Verification items for the finished model (mm, model axes). Face numbers are marked on the shaded views. A direction names the side the tool comes from. Coordinates: 2 decimals unless noted, no trailing zeros. Loops run counter-clockwise (first coordinate to the right, second up) from the corner with the lowest first, then second, coordinate; pieces in that order, holes last. Notation, with made-up numbers: (20, -32) -> (71, -32) arc R31 ccw to (71, -4) -> close; hole circle Ø8 at (42, 53.5). An arc over 180 degrees is marked (long way). Write item = value, one per line.
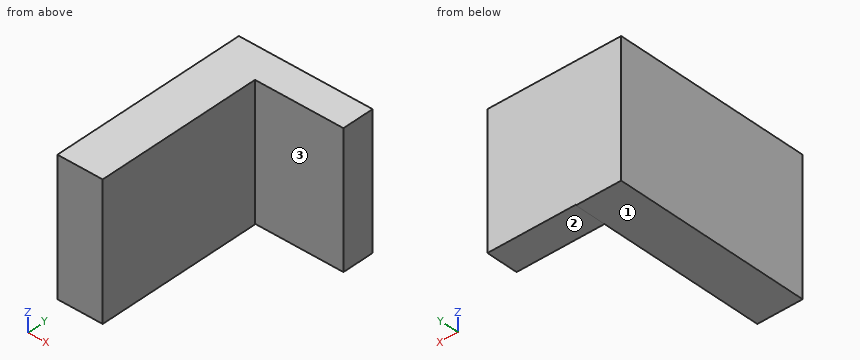
```python
from build123d import *

# Parameters (mm, degrees)
F0_W     = 41.935582
F0_H     = 41.549082
F1_DEPTH = 10
F3_DEPTH = 14.2


with BuildPart() as f1:
    # F0 (on Front) → F1 (new body)
    with BuildSketch(Plane.XZ):
        with Locations((-43.771474, 27.44172)):
            Rectangle(F0_W, F0_H)
    extrude(amount=F1_DEPTH)

    # F2 (on face) → F3 (join)
    with BuildSketch(Plane(origin=(-64.739265, 0, 0), x_dir=(0, -1, 0), z_dir=(-1, 0, 0))):
        Polygon((62.226996, 48.216261), (10, 48.216261), (10, 6.667179), (0, 6.667179), (0, 6.473927), (62.226996, 6.473927), align=None)
    extrude(amount=-F3_DEPTH)


solid = f1.part
```
1) Sectioned sample at A-A, the plane z = 23. Record the cut outline in (x, y).
Ans:
outline = (-64.74, -62.23) -> (-50.54, -62.23) -> (-50.54, -10) -> (-22.8, -10) -> (-22.8, 0) -> (-64.74, 0) -> close
2) Material ranges on line 1 (X direction, y = -47, z = 44.5); line 2 (Y direction, x = -25.5, z = 27), recorded low to high.
Ans:
line_1 = -64.74 to -50.54
line_2 = -10 to 0
3) Depth check by flat-ended pin: pin 1 Ø12 at (x, y) = (-28, -11) entering from -Z; pin 2 Ø6 at (y, z) = (-43.5, 22) entering from +X; pin 3 Ø1.5 at (x, z) = (-38, 17.5) entering from +Y. Enter the tip coordinate at first touch or a pass-through.
Ans:
pin_1 = 6.67
pin_2 = -50.54
pin_3 = 0
4) Tool access check on the marked faces 1, 2 and 3. Record the directions out of +Z, -Z, +X, -X, +Y, -Y that give a thin tool (end or side, any length) a straight path to the whole face; none if there is none.
Ans:
face_1 = -Z, +X, -X, +Y, -Y
face_2 = -Z, +X, +Y, -Y
face_3 = +Z, -Z, +X, -Y
5) Sectioned sample at B-B, the plane x = -28. Record the cut outline in (y, z), plus the area to 3 significant figures.
Ans:
outline = (-10, 6.67) -> (0, 6.67) -> (0, 48.22) -> (-10, 48.22) -> close
area = 415 mm2
6) Sectioned sample at C-C, the plane y = -21. Record the cut outline in (x, z), plus the area to 3 significant figures.
Ans:
outline = (-64.74, 6.47) -> (-50.54, 6.47) -> (-50.54, 48.22) -> (-64.74, 48.22) -> close
area = 593 mm2
